from build123d import *

# Parameters (mm, degrees)
SKETCH1_W       = 160
SKETCH1_H       = 118.25
MAIN_BODY_DEPTH = 38
TRACK_DEPTH     = 106
FILLET_2_R      = 5
SKETCH3_W       = 139
SKETCH3_H       = 112.25
STORAGE_DEPTH   = 35
WIRE_HOLE_DEPTH = 25
FILLET2_R       = 1
CHAMFER1_SIZE   = 2


with BuildPart() as part:
    # Sketch1 → Main Body (new body)
    with BuildSketch(Plane.XY):
        Rectangle(SKETCH1_W, SKETCH1_H)
    extrude(amount=MAIN_BODY_DEPTH)

    # Sketch2 → Track (add)
    with BuildSketch(Plane.XZ.offset(59.125)):
        Polygon((-72.5, 38), (-74.2, 38), (-74.2, 40.2), (-75.5, 40.2), (-75.5, 42.75), (-69.5, 42.75), (-69.5, 40.2), (-70.8, 40.2), (-70.8, 38), align=None)
    track = extrude(amount=-TRACK_DEPTH)

    # Mirror Track: Track across plane
    add(track.mirror(Plane(origin=(0, 0, 0), x_dir=(0, 0, 1), z_dir=(1, 0, 0))))

    # Fillet 2
    fillet_2_edges = [part.edges().sort_by_distance(p)[0] for p in [
        (-80, 0, 0),
        (0, 59.125, 0),
        (80, 0, 0),
        (-80, 59.125, 19),
        (80, 59.125, 19),
    ]]
    fillet(fillet_2_edges, radius=FILLET_2_R)

    # Sketch3 → Storage (cut)
    with BuildSketch(Plane.XY.offset(38)):
        Rectangle(SKETCH3_W, SKETCH3_H)
    extrude(amount=-STORAGE_DEPTH, mode=Mode.SUBTRACT)

    # Sketch4 → Wire Hole (cut)
    with BuildSketch(Plane.XY.offset(3)):
        with BuildLine():
            Line((-7.5, -36.125), (7.5, -36.125))
            ThreePointArc((7.5, -36.125), (12.5, -41.125), (7.5, -46.125))
            Line((7.5, -46.125), (-7.5, -46.125))
            ThreePointArc((-7.5, -46.125), (-12.5, -41.125), (-7.5, -36.125))
        make_face()
    extrude(amount=-WIRE_HOLE_DEPTH, mode=Mode.SUBTRACT)

    # Fillet2
    fillet2_edges = [part.edges().sort_by_distance(p)[0] for p in [
        (-12.5, -41.125, 0),
        (0, -36.125, 0),
        (12.5, -41.125, 0),
        (0, -46.125, 0),
        (0, -59.125, 38),
    ]]
    fillet(fillet2_edges, radius=FILLET2_R)

    # Chamfer1
    chamfer1_edges = [part.edges().sort_by_distance(p)[0] for p in [
        (0, 56.125, 38),
    ]]
    chamfer(chamfer1_edges, length=CHAMFER1_SIZE)


solid = part.part
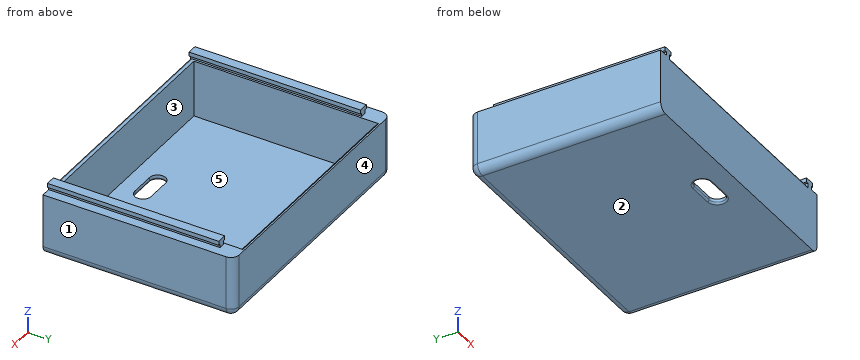
Design review of the part built by this model. Coordinates are the model's own, in mm. Face numbers are marked on the shaded views. A direction names the side the tool comes from. Give positions to 0.01 mm unless a question says otherwise; leave off trailing zeros. Order: outer loops, then holes, each group sorted by start corner. A loop starts at its lowest first (then second) coordinate and runs counter-clockwise, first axis right, second up. Notation, with made-up numbers: (9.5, 9.25) - (59.5, 9.25) arc R8 cw to (59.5, 16.25) - close; hole circle Ø8 at (38, 73). An arc over 180 degrees is marked (long way). Write item = value, one per line. Start each with the question number.
Q1. We need section C-C on x = -23.5. State the section outline as (y, z) points (3 decimals).
Q2. We need section A-A on z = 19. State the section outline as (x, y) points (3 decimals), plus the area to 3 significant figures.
Q3. Mouldability with a two-part tool opening along X and no side actions: class the marked faces 1, 2 and 3 as released by +X, released by -X, zero draft, split by the parting line, or undercut.
Q4. To check wall thickness, follow L1, parallel to Y at x = -33, z = 17.5 (3 decimals); L2, parallel to X at y = 4.5, z = 39; L3, parallel to X at y = 22, z = 10.5. State the ranges of each line that lie inside material, in increasing order. Write a range as from..to.
Q5. Tool access review of the marked faces 4 and 5: name each direction out of +Z, -Z, +X, -X, +Y, -Y from which nothing blocks a thin tool from reaching the whole face with its end or side.
Q6. Clearance check with flat-ended pins moving along their axes: pin 1 Ø1.3 at (y, z) = (3, 41) entering from +X; pin 2 Ø1 at (y, z) = (-32, 39) entering from +X; pin 3 Ø0.6 at (x, z) = (1.5, 1.5) entering from +Y. State where each tip first meets the part, or that it passes through.
Q7. We need section B-B on y = -12. State the section outline as (x, z) points, plus the area to 3 significant figures.
Working result:
q1.outline = (-59.125, 0) - (54.125, 0) arc R5 ccw to (59.125, 5) - (59.125, 38) - (58.125, 38) - (56.125, 36) - (56.125, 3) - (-56.125, 3) - (-56.125, 38) - (-58.125, 38) arc R1 ccw to (-59.125, 37) - close
q2.outline = (-80, -59.125) - (80, -59.125) - (80, 54.125) arc R5 ccw to (75, 59.125) - (-75, 59.125) arc R5 ccw to (-80, 54.125) - close; hole (-69.5, -56.125) - (69.5, -56.125) - (69.5, 56.125) - (-69.5, 56.125) - close
q2.area = 3,310 mm²
q3.face_1 = released by +X
q3.face_2 = zero draft
q3.face_3 = undercut
q4.L1 = -59.125..-56.125, 56.125..59.125
q4.L2 = -74.2..-70.8, 70.8..74.2
q4.L3 = -80..-69.5, 69.5..80
q5.face_4 = +Z, -Z, +X, -X, +Y
q5.face_5 = +Z
q6.pin_1 = 75.5
q6.pin_2 = 74.2
q6.pin_3 = 57.97
q7.outline = (-80, 5) arc R5 ccw to (-75, 0) - (75, 0) arc R5 ccw to (80, 5) - (80, 38) - (74.2, 38) - (74.2, 40.2) - (75.5, 40.2) - (75.5, 42.75) - (69.5, 42.75) - (69.5, 40.2) - (70.8, 40.2) - (70.8, 38) - (69.5, 38) - (69.5, 3) - (-69.5, 3) - (-69.5, 38) - (-70.8, 38) - (-70.8, 40.2) - (-69.5, 40.2) - (-69.5, 42.75) - (-75.5, 42.75) - (-75.5, 40.2) - (-74.2, 40.2) - (-74.2, 38) - (-80, 38) - close
q7.area = 1,250 mm²
